Check sheet for the drawn part. Datum: minimum x, y, z corner. Units: mm. A direction names the side the tool comes from. Give positions to 0.01 mm unless a question says otherwise; leave off trailing zeros. Loops run counter-clockwise (first coordinate to the right, second up) from the corner with the lowest first, then second, coordinate; pieces in that order, holes last. Notation, with made-up numbers: (4, 10.5) - (28, 10.5) arc R24 ccw to (28, 34.5) - close; hole circle Ø10 at (25, 58.25). An arc over 180 degrees is marked (long way). Use one line per item in the form item = value.
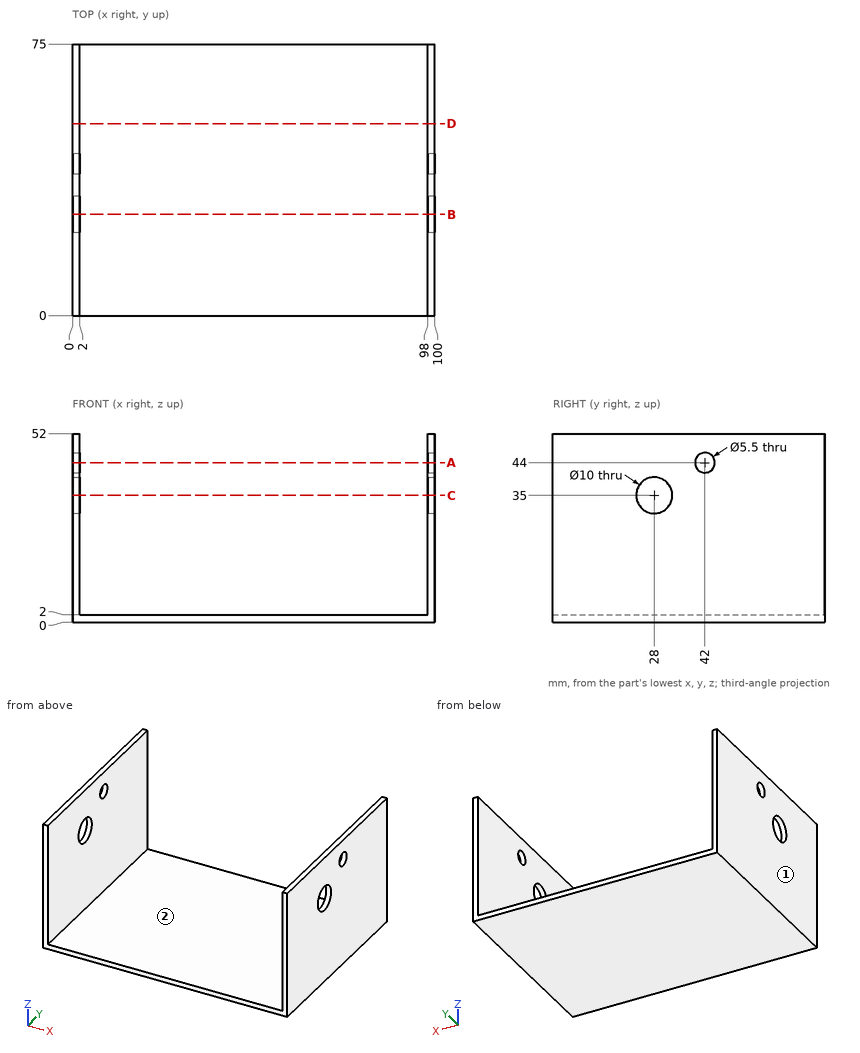
1. Section check C-C, the plane z = 35. Record the cut outline in (x, y).
Result set:
outline = (0, 0) - (2, 0) - (2, 23) - (0, 23) - close; (0, 33) - (2, 33) - (2, 75) - (0, 75) - close; (98, 0) - (100, 0) - (100, 23) - (98, 23) - close; (98, 33) - (100, 33) - (100, 75) - (98, 75) - close
2. Scan lines: probe 1 along X at (y, z) = (62, 32); probe 2 along Z at (x, y) = (99.35, 28); probe 3 along Z at (x, y) = (1, 42). Record each from-to range of solid material in increasing order.
Result set:
probe_1 = 0 to 2, 98 to 100
probe_2 = 0 to 30, 40 to 52
probe_3 = 0 to 41.25, 46.75 to 52
3. Section check B-B, the plane y = 28. Record the cut outline in (x, z), then the cut area to 3 significant figures.
Result set:
outline = (0, 0) - (100, 0) - (100, 30) - (98, 30) - (98, 2) - (2, 2) - (2, 30) - (0, 30) - close; (0, 40) - (2, 40) - (2, 52) - (0, 52) - close; (98, 40) - (100, 40) - (100, 52) - (98, 52) - close
area = 360 mm²
4. Section check A-A, the plane z = 44. Record the cut outline in (x, y), then the cut area to 3 significant figures.
Result set:
outline = (0, 0) - (2, 0) - (2, 39.25) - (0, 39.25) - close; (0, 44.75) - (2, 44.75) - (2, 75) - (0, 75) - close; (98, 0) - (100, 0) - (100, 39.25) - (98, 39.25) - close; (98, 44.75) - (100, 44.75) - (100, 75) - (98, 75) - close
area = 278 mm²
5. Tool access check on the marked faces 1 and 2. Record the directions out of +Z, -Z, +X, -X, +Y, -Y that give a thin tool (end or side, any length) a straight path to the whole face; none if there is none.
Result set:
face_1 = +Z, -Z, -X, +Y, -Y
face_2 = +Z, +Y, -Y
6. Depth check by flat-ended pin: pin 1 Ø4.5 at (y, z) = (42, 44) entering from -X; pin 2 Ø1 at (x, y) = (45.5, 21) entering from +Z. Enter the tip coordinate at first touch or a pass-through.
Result set:
pin_1 = through
pin_2 = 2
7. Section check D-D, the plane y = 53. Record the cut outline in (x, z).
Result set:
outline = (0, 0) - (100, 0) - (100, 52) - (98, 52) - (98, 2) - (2, 2) - (2, 52) - (0, 52) - close
